```python
from build123d import *

# Parameters (mm, degrees)
SKETCH1_R               = 24.60625
SKETCH1_R_2             = 20.32
BOSS_EXTRUDE1_DEPTH     = 95.25
SKETCH2_R               = 28.575
SKETCH2_R_2             = 24.60625
BOSS_EXTRUDE2_DEPTH     = 95.25
SKETCH3_W               = 57.15
SKETCH3_H               = 74.93
CUT_EXTRUDE1_DEPTH      = 29.575
CUT_EXTRUDE1_DEPTH_BACK = 29.575
SKETCH4_R               = 24.60625
SKETCH4_R_2             = 20.32
BOSS_EXTRUDE3_DEPTH     = 74.93


with BuildPart() as part:
    # Sketch1 → Boss-Extrude1 (new body)
    with BuildSketch(Plane(origin=(0, 0, 0), x_dir=(1, 0, 0), z_dir=(0, 1, 0))):
        Circle(SKETCH1_R)
        Circle(SKETCH1_R_2, mode=Mode.SUBTRACT)
    extrude(amount=BOSS_EXTRUDE1_DEPTH)

    # Sketch2 → Boss-Extrude2 (add)
    with BuildSketch(Plane(origin=(0, 95.25, 0), x_dir=(1, 0, 0), z_dir=(0, 1, 0))):
        Circle(SKETCH2_R)
        Circle(SKETCH2_R_2, mode=Mode.SUBTRACT)
    extrude(amount=-BOSS_EXTRUDE2_DEPTH)

    # Sketch3 → Cut-Extrude1 (cut, two sides)
    with BuildSketch(Plane.XY) as cut_extrude1_sk:
        with Locations((0, 47.625)):
            Rectangle(SKETCH3_W, SKETCH3_H)
    extrude(amount=CUT_EXTRUDE1_DEPTH, mode=Mode.SUBTRACT)
    extrude(cut_extrude1_sk.sketch, amount=-CUT_EXTRUDE1_DEPTH_BACK, mode=Mode.SUBTRACT)

    # Sketch4 → Boss-Extrude3 (add)
    with BuildSketch(Plane(origin=(0, 10.16, 0), x_dir=(1, 0, 0), z_dir=(0, 1, 0))):
        Circle(SKETCH4_R)
        Circle(SKETCH4_R_2, mode=Mode.SUBTRACT)
    extrude(amount=BOSS_EXTRUDE3_DEPTH)


solid = part.part
```
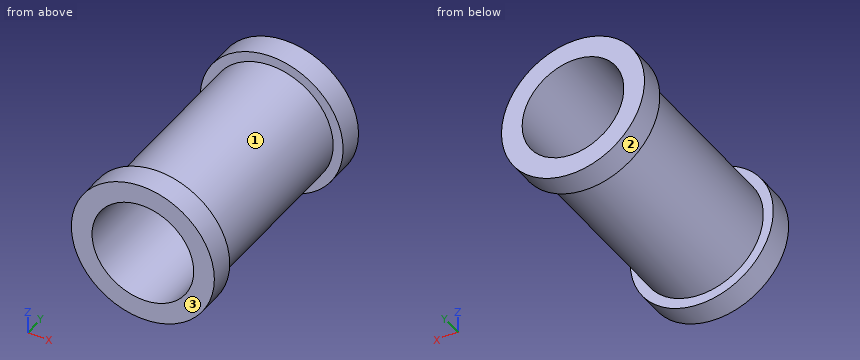
Verification items for the finished model (mm, model axes). Face numbers are marked on the shaded views. Round coordinates to 2 decimals unless told otherwise and drop trailing zeros. Order: outer loops, then holes, each group sorted by start corner. A loop starts at its lowest first (then second) coordinate and runs counter-clockwise, first axis right, second up.
1) Depth check by flat-ended pin: pin 1 (3 mm diameter, centred on y = 13.5, z = -10, fed in from +X); pin 2 (2 mm diameter, centred on x = 4, y = 26, fed in from -Z); pin 3 (8 mm diameter, centred on y = 77, z = 18, fed in from -X). Enter the tip coordinate at first touch or a pass-through.
Geometry says:
pin 1: stops at x = 23.09
pin 2: stops at z = -24.42
pin 3: stops at x = -20.24
2) Draft check along Y on the marked faces 1, 2 and 3. Enter one of: +Y half, -Y half, draft (parallel to the pull), parting line (faces both ways), or undercut.
Geometry says:
face 1: undercut
face 2: draft
face 3: -Y half
3) Material ranges on line 1 (X direction, y = 59, z = 0); line 2 (X direction, y = 16, z = 18), recorded low to high.
Geometry says:
line 1: x = -24.61 to -20.32, 20.32 to 24.61
line 2: x = -16.78 to -9.43, 9.43 to 16.78
4) Cross-section at C-C, the plane y = 81. Record the cut outline in (x, z), plus the area to 3 significant figures.
Geometry says:
outline: circle Ø49.21 at (0, 0); hole circle Ø40.64 at (0, 0)
area: 605 mm2
5) Cross-section at A-A, the plane z = 0. Record the cut outline in (x, y) (3 decimals).
Geometry says:
outline: (-28.575, 0) - (-20.32, 0) - (-20.32, 95.25) - (-28.575, 95.25) - (-28.575, 85.09) - (-24.606, 85.09) - (-24.606, 10.16) - (-28.575, 10.16) - close; (20.32, 0) - (28.575, 0) - (28.575, 10.16) - (24.606, 10.16) - (24.606, 85.09) - (28.575, 85.09) - (28.575, 95.25) - (20.32, 95.25) - close
6) Cross-section at B-B, the plane x = 0. Record the cut outline in (y, z) (3 decimals), plus the area to 3 significant figures.
Geometry says:
outline: (0, -28.575) - (10.16, -28.575) - (10.16, -24.606) - (85.09, -24.606) - (85.09, -28.575) - (95.25, -28.575) - (95.25, -20.32) - (0, -20.32) - close; (0, 20.32) - (95.25, 20.32) - (95.25, 28.575) - (85.09, 28.575) - (85.09, 24.606) - (10.16, 24.606) - (10.16, 28.575) - (0, 28.575) - close
area: 978 mm2
7) Cross-section at D-D, the plane x = -22. Record the cut outline in (y, z).
Geometry says:
outline: (0, -18.24) - (10.16, -18.24) - (10.16, -11.02) - (85.09, -11.02) - (85.09, -18.24) - (95.25, -18.24) - (95.25, 18.24) - (85.09, 18.24) - (85.09, 11.02) - (10.16, 11.02) - (10.16, 18.24) - (0, 18.24) - close
